Could you check a few things on this drawing? It's one solid part, dimensions in mm from its lowest x, y, z. A direction names the side the tool comes from. Round coordinates to 2 decimals unless told otherwise and drop trailing zeros. Write each loop counter-clockwise with the first axis right and the second up, starting at its lowest first coordinate (ties: lowest second). Pieces come first, ordered by that corner, then holes. Notation, with made-up numbers: (6.25, 23.25) - (13.25, 23.25) arc R34 ccw to (13.25, 61.25) - close; hole circle Ø6 at (-26.5, 24.5). An arc over 180 degrees is marked (long way). One line per question, with ' | ' between items. Start each with the question number.
(1) Imagine slicing it at B-B (y = 55.5). Write out the boundary of the cut face in (x, z).
(2) Imagine slicing it at C-C (x = 61.5). Write out the boundary of the cut face in (y, z), plus the area to 3 significant figures.
(3) If I drill on L1, parallel to Y at x = 65, z = 17.5; L2, parallel to X at y = 66, z = 23, over which ranges is the centre line in solid material (lowest first)?
(4) Will these pins go through, and if not, where does the flat tip stop? pin 1 (12 mm diameter, centred on y = 66, z = 21, fed in from -X); pin 2 (3 mm diameter, centred on x = 50, z = 18.5, fed in from +Y).
(5) For the marked faces 1 and 2, which set-ups out of +Z, -Z, +X, -X, +Y, -Y let a thin tool reach every point of the face, with its end or its side?
(6) Imagine slicing it at A-A (z = 8.25). Write out the boundary of the cut face in (x, y), plus the area to 3 significant figures.
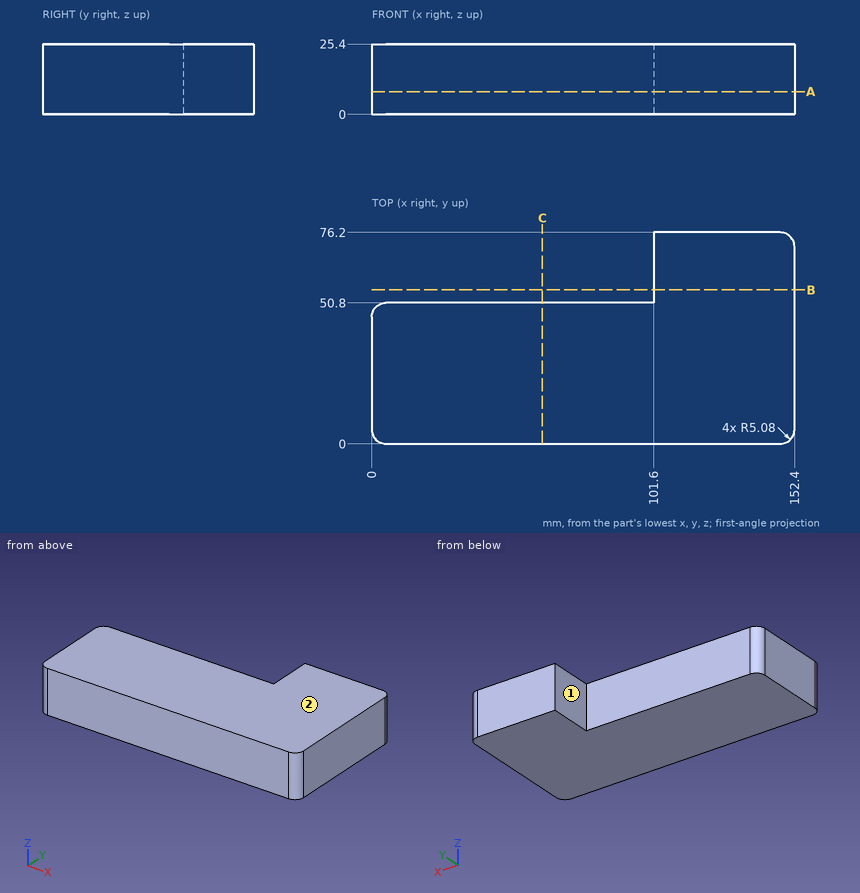
Check sheet entries:
1) outline: (101.6, 0) - (152.4, 0) - (152.4, 25.4) - (101.6, 25.4) - close
2) outline: (0, 0) - (50.8, 0) - (50.8, 25.4) - (0, 25.4) - close | area: 1,290 mm^2
3) L1: 0 to 50.8 | L2: 101.6 to 152.4
4) pin 1: x = 101.6 | pin 2: y = 50.8
5) face 1: +Z, -Z, -X, +Y | face 2: +Z, +X, -X, +Y, -Y
6) outline: (0, 5.08) arc R5.08 ccw to (5.08, 0) - (147.32, 0) arc R5.08 ccw to (152.4, 5.08) - (152.4, 71.12) arc R5.08 ccw to (147.32, 76.2) - (101.6, 76.2) - (101.6, 50.8) - (5.08, 50.8) arc R5.08 ccw to (0, 45.72) - close | area: 9,010 mm^2
